Geometry check sheet. Reference: the model listing, model coordinates, mm. A direction names the side the tool comes from. Round coordinates to 2 decimals unless told otherwise and drop trailing zeros. Loops run counter-clockwise (first coordinate to the right, second up) from the corner with the lowest first, then second, coordinate; pieces in that order, holes last.
```python
from build123d import *

# Parameters (mm, degrees)
F2_DEPTH      = 12.7
F2_DEPTH_BACK = 12.7
F1_R          = 14.6016547105
F3_DEPTH      = 12.7
F3_DEPTH_BACK = 12.7


with BuildPart() as f2:
    # F0 (on Front) → F2 (new body, two sides)
    with BuildSketch(Plane.XZ) as f2_sk:
        with BuildLine():
            Line((12.7, 34.4253193842), (0, 34.4253193842))
            Line((0, 34.4253193842), (0, -5.8595561422))
            Line((0, -5.8595561422), (0, -6.2146806158))
            Line((0, -6.2146806158), (19.245794032, -6.2146806158))
            Line((19.245794032, -6.2146806158), (38.1, -6.2146806158))
            Line((38.1, -6.2146806158), (38.1, 9.0253193842))
            ThreePointArc((38.1, 9.0253193842), (30.6605122421, 26.9858316263), (12.7, 34.4253193842))
        make_face()
        with BuildLine():
            Line((0, -5.8595561422), (0, 34.4253193842))
            Line((0, 34.4253193842), (-12.7, 34.4253193842))
            ThreePointArc((-12.7, 34.4253193842), (-30.6605122421, 26.9858316263), (-38.1, 9.0253193842))
            Line((-38.1, 9.0253193842), (-38.1, -6.2146806158))
            Line((-38.1, -6.2146806158), (-19.245794032, -6.2146806158))
            Line((-19.245794032, -6.2146806158), (0, -5.8595561422))
        make_face()
        Polygon((0, -6.2146806158), (0, -5.8595561422), (-19.245794032, -6.2146806158), align=None)
        Polygon((19.245794032, -6.2146806158), (0, -6.2146806158), (-19.245794032, -6.2146806158), (-7.6351859607, -44.2130304873), (7.6351859607, -44.2130304873), align=None)
    extrude(amount=F2_DEPTH)
    extrude(f2_sk.sketch, amount=-F2_DEPTH_BACK)

    # F1 (on Front) → F3 (join, two sides)
    with BuildSketch(Plane.XZ) as f3_sk:
        with Locations((0, 48.4745278955)):
            Circle(F1_R)
    extrude(amount=F3_DEPTH)
    extrude(f3_sk.sketch, amount=-F3_DEPTH_BACK)


solid = f2.part
```
1) Scan lines: line 1 along X through (y, z) = (9, 9.5); line 2 along X through (y, z) = (-10.5, -38); line 3 along Z through (x, y) = (23, 0.5). Record each from-to range of solid material in increasing order.
Report:
line 1: x = -38.1 to 38.1
line 2: x = -9.53 to 9.53
line 3: z = -6.21 to 32.24
2) Sectioned sample at A-A, the plane y = 9.5. Record the cut outline in (x, z).
Report:
outline: (-38.1, -6.21) - (-19.25, -6.21) - (-7.64, -44.21) - (7.64, -44.21) - (19.25, -6.21) - (38.1, -6.21) - (38.1, 9.03) arc R25.4 ccw to (12.7, 34.43) - (3.98, 34.43) arc R14.6 ccw (long way) to (-3.98, 34.43) - (-12.7, 34.43) arc R25.4 ccw to (-38.1, 9.03) - close
3) Mould release check, pull along Z, two halves, no side actions. Record for faces 1 (the face through (8, 0, 34.425)), 2 (the face through (-13.52, -0.18, -24.95)), 3 (the face through (-1, 12.7, 10)): +Z half, -Z half, draft (parallel to the pull), parting line (faces both ways), or undercut.
Report:
face 1: undercut
face 2: -Z half
face 3: draft
4) Sectioned sample at B-B, the plane x = -28. Record the cut outline in (y, z).
Report:
outline: (-12.7, -6.21) - (12.7, -6.21) - (12.7, 29.3) - (-12.7, 29.3) - close
5) Access from +Z, -Z, +X, -X, +Y, -Y to the whole of each face (thin tool, end or side, straight path). Record for faces 4 (the face through (0, 0, -44.213)), 5 (the face through (29, 0, -6.215)), 6 (the face through (-29, 0, -6.215)).
Report:
face 4: -Z, +X, -X, +Y, -Y
face 5: -Z, +X, +Y, -Y
face 6: -Z, -X, +Y, -Y
6) Sectioned sample at C-C, the plane z = 22. Record the cut outline in (x, y), then the cut area to 3 significant figures.
Report:
outline: (-34.54, -12.7) - (34.54, -12.7) - (34.54, 12.7) - (-34.54, 12.7) - close
area: 1,750 mm2
7) Gauge pin test, flat ends, axial feed: pin 1 (4.5 mm diameter, centred on x = 7, y = 5, fed in from +Z); pin 2 (7 mm diameter, centred on x = -10, y = -3, fed in from +Z); pin 3 (9.5 mm diameter, centred on x = -32.5, y = 4, fed in from -Z); pin 4 (2 mm diameter, centred on x = 29, z = 31, fed in from -Y) (3 decimals). Record the tip position at first contact, or that the pin passes through.
Report:
pin 1: stops at z = 62.28
pin 2: stops at z = 61.55
pin 3: stops at z = -6.21
pin 4: passes through
